```python
from build123d import *
from build123d.topology import SkipClean

# Parameters (mm, degrees)
SKETCH1_R           = 4.85
SKETCH1_R_2         = 2
BOSS_EXTRUDE1_DEPTH = 9
BOSS_EXTRUDE2_DEPTH = 8
SKETCH4_R           = 2
CUT_EXTRUDE1_DEPTH  = 10
SKETCH5_R           = 2
CUT_EXTRUDE2_DEPTH  = 10


with BuildPart() as part:
    # Sketch1 → Boss-Extrude1 (new body)
    with BuildSketch(Plane(origin=(0, 0, 0), x_dir=(1, 0, 0), z_dir=(0, 1, 0))):
        with Locations(Location((0, 0, 0), (0, 0, 270))):
            Circle(SKETCH1_R)
        with Locations(Location((0, 0, 0), (0, 0, 270))):
            Circle(SKETCH1_R_2, mode=Mode.SUBTRACT)
    extrude(amount=BOSS_EXTRUDE1_DEPTH)

    # Sketch2 → Boss-Extrude2 (add)
    with SkipClean():  # the faces are left unmerged after this step: merging them gives an invalid solid
        with BuildSketch(Plane(origin=(0, 9, 0), x_dir=(1, 0, 0), z_dir=(0, 1, 0))):
            with BuildLine():
                Line((-4.85, 0), (-4.85, 70))
                ThreePointArc((-4.85, 70), (0, 74.85), (4.85, 70))
                Line((4.85, 70), (4.85, 0))
                ThreePointArc((4.85, 0), (0, -4.85), (-4.85, 0))
            make_face()
        extrude(amount=BOSS_EXTRUDE2_DEPTH)
    add(part.part.scale(1), mode=Mode.REPLACE)  # the faces are merged on a copy

    # Sketch4 → Cut-Extrude1 (cut)
    with BuildSketch(Plane.XZ.offset(-9)):
        with Locations(Location((0, 0, 0), (0, 0, 90))):
            Circle(SKETCH4_R)
    extrude(amount=-CUT_EXTRUDE1_DEPTH, mode=Mode.SUBTRACT)

    # Sketch5 → Cut-Extrude2 (cut)
    with BuildSketch(Plane(origin=(0, 17, 0), x_dir=(1, 0, 0), z_dir=(0, 1, 0))):
        with Locations(Location((-0.15, 69.852250506, 0), (0, 0, 270))):
            Circle(SKETCH5_R)
    extrude(amount=-CUT_EXTRUDE2_DEPTH, mode=Mode.SUBTRACT)


solid = part.part
```
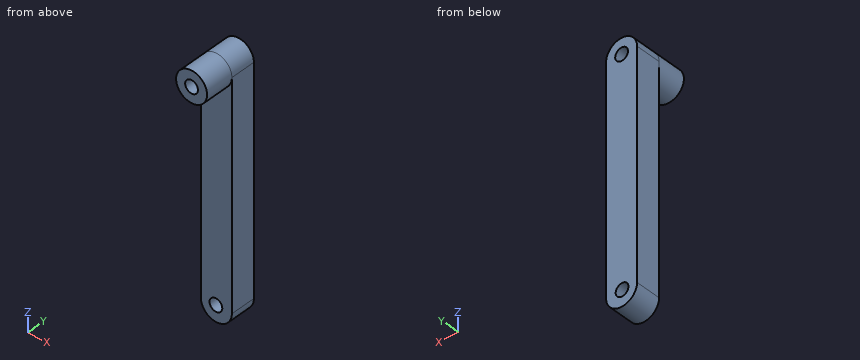
Geometry: final body of the model. Coordinates: model frame, mm. Round coordinates to 2 decimals unless told otherwise and drop trailing zeros. Write each loop counter-clockwise with the first axis right and the second up, starting at its lowest first coordinate (ties: lowest second). Pieces come first, ordered by that corner, then holes.
Item 1: Section query C-C (y = 14.75). Return loops of the section in (x, z).
Item 2: Section query B-B (x = 0.75). Return loops of the section in (y, z).
Item 3: Pin query (flat end, axial travel): P1, Ø6, axis at y = 4, z = -38, coming from the -X side; P2, Ø4, axis at x = 1.5, z = -53.5, coming from the -Y side; P3, Ø1.5, axis at x = 2, y = 3, coming from the +Z side; P4, Ø5, axis at x = 3, y = 6, coming from the +Z side. Return the tip coordinate at first contact, or that it passes through.
Item 4: Material intervals for L1, parallel to Z at x = 0, y = 12; L2, parallel to Y at x = 0, z = -56; L3, parallel to Z at x = -1.5, y = 15.25, sorted ascending.
Item 5: Section query D-D (z = -42). Return loops of the section in (x, y), plus the area to 3 significant figures.
Item 6: Section query A-A (y = 3.5). Return loops of the section in (x, z), plus the area to 3 significant figures.
Completed:
1. outline: (-4.85, -70) arc R4.85 ccw to (4.85, -70) - (4.85, 0) arc R4.85 ccw to (-4.85, 0) - close; hole circle Ø4 at (-0.15, -69.85); hole circle Ø4 at (0, 0)
2. outline: (0, -4.79) - (9, -4.79) - (9, -68.07) - (17, -68.07) - (17, -1.85) - (0, -1.85) - close; (0, 1.85) - (17, 1.85) - (17, 4.79) - (0, 4.79) - close; (9, -74.79) - (17, -74.79) - (17, -71.64) - (9, -71.64) - close
3. P1: passes through
3. P2: stops at y = 9
3. P3: stops at z = 4.69
3. P4: stops at z = 4.82
4. L1: z = -74.85 to -71.85, -67.86 to -2, 2 to 4.85
4. L2: y = 9 to 17
4. L3: z = -74.61 to -71.33, -68.38 to -1.32, 1.32 to 4.61
5. outline: (-4.85, 9) - (4.85, 9) - (4.85, 17) - (-4.85, 17) - close
5. area: 77.6 mm2
6. outline: circle Ø9.7 at (0, 0); hole circle Ø4 at (0, 0)
6. area: 61.3 mm2
